Work out the finished part from the listing and answer in its coordinate system (mm). Face numbers are marked on the shaded views. Give positions to 0.01 mm unless a question says otherwise; leave off trailing zeros. Order: outer loops, then holes, each group sorted by start corner. A loop starts at its lowest first (then second) coordinate and runs counter-clockwise, first axis right, second up. Notation, with made-up numbers: (5, 41) - (48, 41) arc R24 ccw to (48, 56) - close; hole circle Ø10 at (85, 74). An arc over 180 degrees is marked (long way). Put each result on its own line as item: value.
```python
from build123d import *

# Parameters (mm, degrees)
SKETCH1_R           = 4
SKETCH1_R_2         = 2.5
BOSS_EXTRUDE1_DEPTH = 11
SKETCH2_R           = 4
BOSS_EXTRUDE2_DEPTH = 5


with BuildPart() as part:
    # Sketch1 → Boss-Extrude1 (new body)
    with BuildSketch(Plane(origin=(0, 0, 0), x_dir=(1, 0, 0), z_dir=(0, 1, 0))):
        with Locations(Location((0, 0, 0), (0, 0, 270))):
            Circle(SKETCH1_R)
        with Locations(Location((0, 0, 0), (0, 0, 270))):
            Circle(SKETCH1_R_2, mode=Mode.SUBTRACT)
    extrude(amount=BOSS_EXTRUDE1_DEPTH)

    # Sketch2 → Boss-Extrude2 (add)
    with BuildSketch(Plane(origin=(0, 11, 0), x_dir=(1, 0, 0), z_dir=(0, 1, 0))):
        with Locations(Location((0, 0, 0), (0, 0, 270))):
            Circle(SKETCH2_R)
        with BuildLine():
            Line((1.920937271, 1.6), (-1.920937271, 1.6))
            ThreePointArc((-1.920937271, 1.6), (-2.5, 0), (-1.920937271, -1.6))
            Line((-1.920937271, -1.6), (1.920937271, -1.6))
            ThreePointArc((1.920937271, -1.6), (2.5, 0), (1.920937271, 1.6))
        make_face(mode=Mode.SUBTRACT)
    extrude(amount=BOSS_EXTRUDE2_DEPTH)


solid = part.part
```
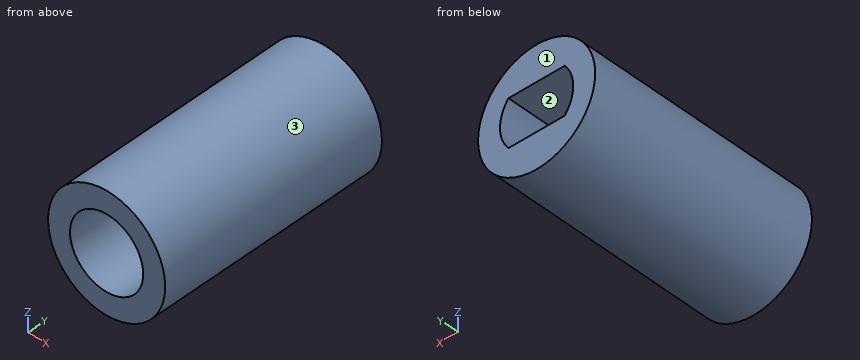
(1) Section A-A, the plane z = 0 is taken. Write down the section's boundary in (x, y).
Geometry check:
outline: (-4, 0) - (-2.5, 0) - (-2.5, 16) - (-4, 16) - close; (2.5, 0) - (4, 0) - (4, 16) - (2.5, 16) - close
(2) Section C-C, the plane y = 14.5 is taken. Write down the section's boundary in (x, z), then the cut area to 3 significant figures.
Geometry check:
outline: circle Ø8 at (0, 0); hole (-1.92, -1.6) - (1.92, -1.6) arc R2.5 ccw to (1.92, 1.6) - (-1.92, 1.6) arc R2.5 ccw to start
area: 35.4 mm²
(3) Given pin 1 (0.7 mm diameter, centred on x = 0, z = -2, fed in from -Y); pin 2 (4 mm diameter, centred on x = -0.5, y = 14, fed in from -Z); pin 3 (1 mm diameter, centred on y = 8, z = 1.5, fed in from -X); pin 4 (3 mm diameter, centred on x = 0, z = 0, fed in from -Y), each flat-ended and moving along its own axis, determine where each tip first touches the part or whether it passes through.
Geometry check:
pin 1: stops at y = 11
pin 2: stops at z = -4
pin 3: stops at x = -3.87
pin 4: passes through
(4) Section B-B, the plane x = 0 is taken. Write down the section's boundary in (y, z).
Geometry check:
outline: (0, -4) - (16, -4) - (16, -1.6) - (11, -1.6) - (11, -2.5) - (0, -2.5) - close; (0, 2.5) - (11, 2.5) - (11, 1.6) - (16, 1.6) - (16, 4) - (0, 4) - close
(5) Straight lines are drawn through the part: line 1 (X direction, y = 8.25, z = 0); line 2 (Y direction, x = 0, z = -2); line 3 (Z direction, x = -1, y = 9.5). For each, find the intervals that lie inside material, in ascending order.
Geometry check:
line 1: x = -4 to -2.5, 2.5 to 4
line 2: y = 11 to 16
line 3: z = -3.87 to -2.29, 2.29 to 3.87
(6) Determine the mould class of the marked faces 1, 2 and 3 for opening direction X: pulls with the +X half, pulls with the -X half, needs draft (parallel to the pull), parting line crosses it, or undercut.
Geometry check:
face 1: needs draft
face 2: undercut
face 3: parting line crosses it
(7) Section D-D, the plane z = 2.25 is taken. Write down the section's boundary in (x, y), then the cut area to 3 significant figures.
Geometry check:
outline: (-3.31, 0) - (-1.09, 0) - (-1.09, 11) - (1.09, 11) - (1.09, 0) - (3.31, 0) - (3.31, 16) - (-3.31, 16) - close
area: 81.9 mm²
